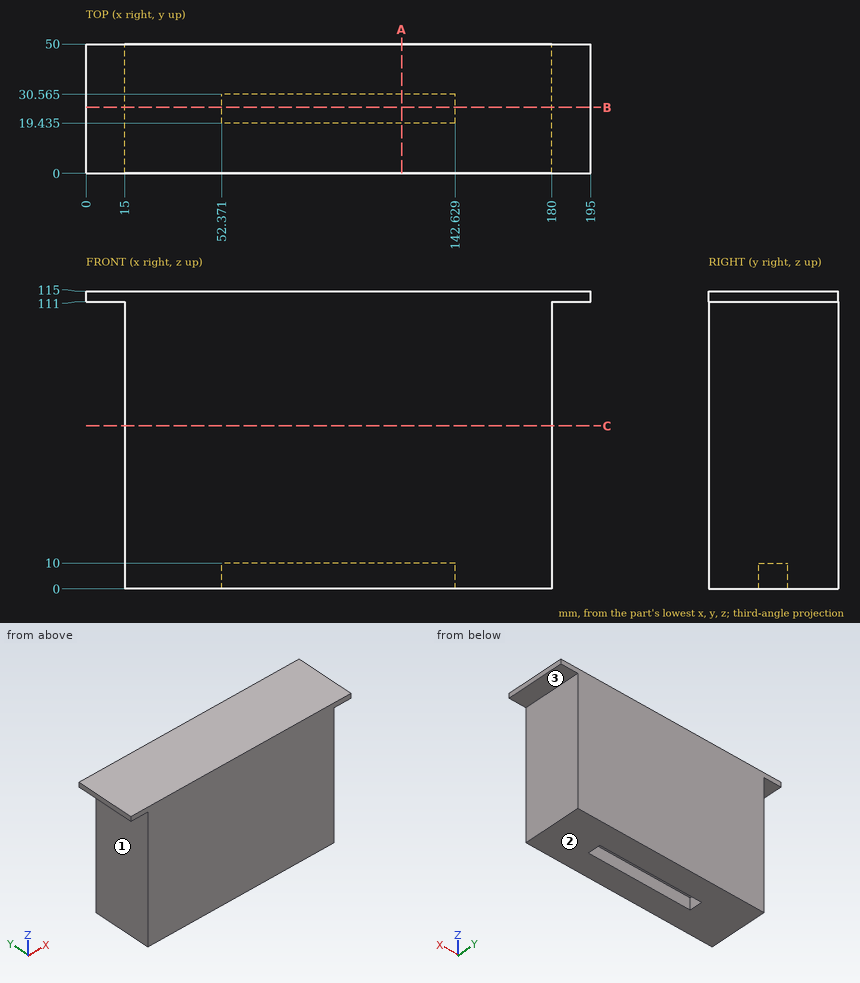
Here's the drawing with two shaded views (mm, measured from the low corner). I have some questions. A direction names the side the tool comes from. Give positions to 0.01 mm unless a question says otherwise; leave off trailing zeros. Loops run counter-clockwise (first coordinate to the right, second up) from the corner with the lowest first, then second, coordinate; pieces in that order, holes last. Notation, with made-up numbers: (-11, 73.5) -> (10, 73.5) arc R29 cw to (10, 99.5) -> close; hole circle Ø7 at (65, 71.25). An arc over 180 degrees is marked (long way). Use one line per item in the form item = value.
1) If we section it at B-B (y = 25.5): Please give me the cut outline in (x, z).
Answers:
outline = (0, 111) -> (15, 111) -> (15, 0) -> (52.37, 0) -> (52.37, 10) -> (142.63, 10) -> (142.63, 0) -> (180, 0) -> (180, 111) -> (195, 111) -> (195, 115) -> (0, 115) -> close
2) I need wall thicknesses on line 1 along X through (y, z) = (28, 9); line 2 along X through (y, z) = (47, 14); line 3 along Z through (x, y) = (125, 20.5). Which ranges of each line are inside material? Lowest first, please.
Answers:
line_1 = 15 to 52.37, 142.63 to 180
line_2 = 15 to 180
line_3 = 10 to 115
3) If we section it at A-A (x = 122): Please give me the cut outline in (y, z) (1 decimal), plus the area to 3 significant figures.
Answers:
outline = (0, 0) -> (19.4, 0) -> (19.4, 10) -> (30.6, 10) -> (30.6, 0) -> (50, 0) -> (50, 115) -> (0, 115) -> close
area = 5,640 mm²
4) Will these pins go through, and if not, where does the flat tip stop? pin 1 (25 mm diameter, centred on y = 33, z = 47, fed in from +X); pin 2 (11 mm diameter, centred on y = 23, z = 5.5, fed in from -X); pin 3 (4.5 mm diameter, centred on x = 187.5, y = 27, fed in from -Z).
Answers:
pin_1 = 180
pin_2 = 15
pin_3 = 111
5) For the marked faces 1, 2 and 3, which set-ups out of +Z, -Z, +X, -X, +Y, -Y let a thin tool reach every point of the face, with its end or its side?
Answers:
face_1 = -Z, -X, +Y, -Y
face_2 = -Z, +X, -X, +Y, -Y
face_3 = -Z, +X, +Y, -Y
6) If we section it at C-C (z = 63): Please give me the cut outline in (x, y).
Answers:
outline = (15, 0) -> (180, 0) -> (180, 50) -> (15, 50) -> close
